```python
from build123d import *

# Parameters (mm, degrees)
F0_R     = 10
F0_R_2   = 8.75
F0_R_3   = 3.95
F1_DEPTH = 14.6
F2_DEPTH = 0.5


with BuildPart() as f1:
    # F0 (on Top) → F1 (new body)
    with BuildSketch(Plane.XY):
        Circle(F0_R)
        Circle(F0_R_2, mode=Mode.SUBTRACT)
        Circle(F0_R_2)
        Circle(F0_R_3, mode=Mode.SUBTRACT)
        Circle(F0_R_3)
    extrude(amount=-F1_DEPTH)

    # F0 (on Top) → F2 (join)
    with BuildSketch(Plane.XY):
        Circle(F0_R)
        Circle(F0_R_2, mode=Mode.SUBTRACT)
        Circle(F0_R_3)
    extrude(amount=F2_DEPTH)


solid = f1.part
```
Geometry check sheet. Reference: the model listing, model coordinates, mm. A direction names the side the tool comes from. Round coordinates to 2 decimals unless told otherwise and drop trailing zeros. Loops run counter-clockwise (first coordinate to the right, second up) from the corner with the lowest first, then second, coordinate; pieces in that order, holes last. Notation, with made-up numbers: (46, 35) -> (86, 35) arc R7 ccw to (86, 43) -> close; hole circle Ø5 at (6, 76). An arc over 180 degrees is marked (long way). Use a Markdown table: item, result.
(1) Sectioned sample at D-D (x = 6.5). Enter the section's corners in (y, z), then the cut area to 3 significant figures.
Calculated:
| item | result |
|---|---|
| outline | (-7.6, -14.6) -> (7.6, -14.6) -> (7.6, 0.5) -> (5.86, 0.5) -> (5.86, 0) -> (-5.86, 0) -> (-5.86, 0.5) -> (-7.6, 0.5) -> close |
| area | 224 mm² |
(2) Go/stop test with flat-tipped pins: P1, Ø4, axis at y = -6.5, z = -2.5, coming from the +X side; P2, Ø6, axis at y = -3.5, z = -12, coming from the -X side. Record where each tip stops, or that it passes through.
Calculated:
| item | result |
|---|---|
| P1 | x = 8.93 |
| P2 | x = -9.99 |
(3) Mould release check, pull along X, two halves, no side actions. Record for faces 3 (the cylindrical face through (-6.944, -5.324, 0.246)), 4 (the flat face through (0, 0, 0.5)), 5 (the cylindrical face through (-3.135, -2.404, 0.246)): released by +X, released by -X, zero draft, split by the parting line, or undercut.
Calculated:
| item | result |
|---|---|
| face 3 | undercut |
| face 4 | zero draft |
| face 5 | undercut |
(4) Sectioned sample at A-A (x = 0). Enter the section's corners in (y, z).
Calculated:
| item | result |
|---|---|
| outline | (-10, -14.6) -> (10, -14.6) -> (10, 0.5) -> (8.75, 0.5) -> (8.75, 0) -> (3.95, 0) -> (3.95, 0.5) -> (-3.95, 0.5) -> (-3.95, 0) -> (-8.75, 0) -> (-8.75, 0.5) -> (-10, 0.5) -> close |
(5) Sectioned sample at C-C (z = -12.75). Enter the section's corners in (x, y).
Calculated:
| item | result |
|---|---|
| outline | circle Ø20 at (0, 0) |
(6) Set-up check for faces 1 (the flat face through (2, -4, 0)), 2 (the flat face through (0, 0, -14.6)): record each of +Z, -Z, +X, -X, +Y, -Y from which the full face is reachable in a straight line by a thin tool's end or side.
Calculated:
| item | result |
|---|---|
| face 1 | +Z |
| face 2 | -Z, +X, -X, +Y, -Y |
(7) Scan lines: probe 1 along Y at (x, z) = (0, 0.3); probe 2 along Z at (x, y) = (-1.25, 7); probe 3 along Y at (x, z) = (0.25, -10.5). Record each from-to range of solid material in increasing order.
Calculated:
| item | result |
|---|---|
| probe 1 | -10 to -8.75, -3.95 to 3.95, 8.75 to 10 |
| probe 2 | -14.6 to 0 |
| probe 3 | -10 to 10 |
